```python
from build123d import *

# Parameters (mm, degrees)
SKETCH1_W           = 31.646470679
SKETCH1_H           = 16.00939105
BOSS_EXTRUDE1_DEPTH = 5
SKETCH1_3_W         = 65
SKETCH1_3_H         = 2.5
BOSS_EXTRUDE2_DEPTH = 20
SKETCH2_W           = 65
SKETCH2_H           = 2.5
BOSS_EXTRUDE3_DEPTH = 5
SKETCH2_3_W         = 65
SKETCH2_3_H         = 2.5
BOSS_EXTRUDE4_DEPTH = 7
SKETCH1_5_W         = 31.646470679
SKETCH1_5_H         = 16.00939105
BOSS_EXTRUDE5_DEPTH = 23
BOSS_EXTRUDE6_DEPTH = 16
BOSS_EXTRUDE7_DEPTH = 2
SKETCH5_W           = 9
SKETCH5_H           = 25
SKETCH5_W_2         = 5
SKETCH5_H_2         = 13.8


with BuildPart() as part:
    # Sketch1 → Boss-Extrude1 (new body)
    with BuildSketch(Plane.XY):
        with BuildLine():
            ThreePointArc((60, 43.75), (63.535533906, 42.285533906), (65, 38.75))
            Line((65, 38.75), (65, 7.5))
            Line((65, 7.5), (0, 7.5))
            Line((0, 7.5), (0, 38.75))
            ThreePointArc((0, 38.75), (1.464466094, 42.285533906), (5, 43.75))
            Line((5, 43.75), (60, 43.75))
        make_face()
        with Locations((31.682365604, 25.44274044)):
            Rectangle(SKETCH1_W, SKETCH1_H, mode=Mode.SUBTRACT)
        with Locations((31.682365604, 25.44274044)):
            Rectangle(SKETCH1_W, SKETCH1_H)
    extrude(amount=BOSS_EXTRUDE1_DEPTH)

    # Sketch1_3 → Boss-Extrude2 (add)
    with BuildSketch(Plane.XY):
        with Locations((32.5, 6.25)):
            Rectangle(SKETCH1_3_W, SKETCH1_3_H)
    extrude(amount=BOSS_EXTRUDE2_DEPTH)

    # Sketch2 → Boss-Extrude3 (add, symmetric)
    with BuildSketch(Plane.XY.offset(10)):
        with Locations((32.5, 3.75)):
            Rectangle(SKETCH2_W, SKETCH2_H)
    extrude(amount=BOSS_EXTRUDE3_DEPTH, both=True)

    # Sketch2_3 → Boss-Extrude4 (add, symmetric)
    with BuildSketch(Plane.XY.offset(10)):
        with Locations((32.5, 1.25)):
            Rectangle(SKETCH2_3_W, SKETCH2_3_H)
    extrude(amount=BOSS_EXTRUDE4_DEPTH, both=True)

    # Sketch1_5 → Boss-Extrude5 (add)
    with BuildSketch(Plane.XY):
        with Locations((31.682365604, 25.44274044)):
            Rectangle(SKETCH1_5_W, SKETCH1_5_H)
    extrude(amount=BOSS_EXTRUDE5_DEPTH)

    # Sketch3 → Boss-Extrude6 (add)
    with BuildSketch(Plane(origin=(0, 0, 0), x_dir=(-1, 0, 0), z_dir=(0, 0, -1))):
        with BuildLine():
            Line((-2, 33.67400262), (0, 33.67400262))
            Line((0, 33.67400262), (0, 38.75))
            ThreePointArc((0, 38.75), (-1.464466094, 42.285533906), (-5, 43.75))
            Line((-5, 43.75), (-60, 43.75))
            ThreePointArc((-60, 43.75), (-63.535533906, 42.285533906), (-65, 38.75))
            Line((-65, 38.75), (-65, 33.551986264))
            Line((-65, 33.551986264), (-63, 33.551986264))
            Line((-63, 33.551986264), (-63, 38.75))
            ThreePointArc((-63, 38.75), (-62.121320344, 40.871320344), (-60, 41.75))
            Line((-60, 41.75), (-5, 41.75))
            ThreePointArc((-5, 41.75), (-2.878679656, 40.871320344), (-2, 38.75))
            Line((-2, 38.75), (-2, 33.67400262))
        make_face()
        Polygon((-9.704230369, -9.009552441), (-4.852115184, -4.157437257), (-6.266328747, -2.743223694), (-10.532657494, -7.009552441), (-53.41460101, -7.009552441), (-57.531707428, -2.550119806), (-58.947047068, -3.965459446), (-54.290161463, -9.009552441), align=None)
    extrude(amount=BOSS_EXTRUDE6_DEPTH)


with BuildPart() as boss_extrude6_piece_1:
    # of the separate pieces the step leaves, piece 1, a body of its own (boss_extrude6_pieces)
    add(part.part.solids().sort_by_distance((65, 0, 3))[0])



with BuildPart() as boss_extrude6_piece_2:
    # of the separate pieces the step leaves, piece 2, a body of its own (boss_extrude6_pieces)
    add(part.part.solids().sort_by_distance((58.947047068, -3.965459446, 0))[0])


with BuildPart() as boss_extrude6_piece_1_1:
    add(boss_extrude6_piece_1.part)

    add(boss_extrude6_piece_2.part)  # Boss-Extrude7 merges Boss-Extrude6 piece 2
    # Sketch4 → Boss-Extrude7 (add)
    with BuildSketch(Plane(origin=(0, 0, -16), x_dir=(-1, 0, 0), z_dir=(0, 0, -1))):
        with BuildLine():
            Line((-60, 41.75), (-5, 41.75))
            ThreePointArc((-5, 41.75), (-2.878679656, 40.871320344), (-2, 38.75))
            Line((-2, 38.75), (-2, 33.67400262))
            Line((-2, 33.67400262), (0, 33.67400262))
            Line((0, 33.67400262), (0, 38.75))
            ThreePointArc((0, 38.75), (-1.464466094, 42.285533906), (-5, 43.75))
            Line((-5, 43.75), (-60, 43.75))
            ThreePointArc((-60, 43.75), (-63.535533906, 42.285533906), (-65, 38.75))
            Line((-65, 38.75), (-65, 33.551986264))
            Line((-65, 33.551986264), (-63, 33.551986264))
            Line((-63, 33.551986264), (-63, 38.75))
            ThreePointArc((-63, 38.75), (-62.121320344, 40.871320344), (-60, 41.75))
        make_face()
        with BuildLine():
            Line((-54.290161463, -9.009552441), (-9.704230369, -9.009552441))
            Line((-9.704230369, -9.009552441), (-4.852115184, -4.157437257))
            Line((-4.852115184, -4.157437257), (0, 0.694677928))
            Line((0, 0.694677928), (0, 33.67400262))
            Line((0, 33.67400262), (-2, 33.67400262))
            Line((-2, 33.67400262), (-2, 38.75))
            ThreePointArc((-2, 38.75), (-2.878679656, 40.871320344), (-5, 41.75))
            Line((-5, 41.75), (-60, 41.75))
            ThreePointArc((-60, 41.75), (-62.121320344, 40.871320344), (-63, 38.75))
            Line((-63, 38.75), (-63, 33.551986264))
            Line((-63, 33.551986264), (-65, 33.551986264))
            Line((-65, 33.551986264), (-65, 2.590780084))
            Line((-65, 2.590780084), (-58.947047068, -3.965459446))
            Line((-58.947047068, -3.965459446), (-54.290161463, -9.009552441))
        make_face()
    extrude(amount=BOSS_EXTRUDE7_DEPTH)

    # Sketch5 → Revolve1 (revolve)
    with BuildSketch(Plane.XY.offset(-6.5)):
        with Locations((28, 78.45)):
            Rectangle(SKETCH5_W, SKETCH5_H)
        Polygon((32.5, 57.55), (32.5, 65.95), (23.5, 65.95), (20.5, 65.95), (20.5, 57.55), (27.5, 57.55), align=None)
        with Locations((30, 50.65)):
            Rectangle(SKETCH5_W_2, SKETCH5_H_2)
    revolve(axis=Axis((32.5, 92.408225654, -6.5), (0, -1, 0)))


solid = boss_extrude6_piece_1_1.part
```
Part model, mm, in its own coordinate system. A direction names the side the tool comes from. Round coordinates to 2 decimals unless told otherwise and drop trailing zeros. Loops run counter-clockwise (first coordinate to the right, second up) from the corner with the lowest first, then second, coordinate; pieces in that order, holes last.
1. Drill centre lines: line 1 along Y through (x, z) = (53, -7); line 2 along Z through (x, y) = (29, 6); line 3 along Z through (x, y) = (6.5, 11.5). Where is each one in solid material? Low to high.
Solutions:
line 1: y = -9.01 to -7.01, 41.75 to 43.75
line 2: z = -18 to -16, 0 to 20
line 3: z = -18 to -16, 0 to 5
2. Two-plate mould, pull along Y, no slides. Class faces 5 (the face through (65, 21, 1)), 6 (the face through (33, 90.95, -7)), 7 (the face through (32, 5, 2)), 8 (the face through (55.444, -4.811, -7.888)): pulls with the +Y half, pulls with the -Y half, needs draft (parallel to the pull), parting line crosses it, or undercut.
Solutions:
face 5: needs draft
face 6: pulls with the +Y half
face 7: undercut
face 8: undercut
3. Slice it at C-C (y = 67). Give the cut face in (x, z), and give its area (3 significant figures).
Solutions:
outline: circle Ø18 at (32.5, -6.5)
area: 254 mm2
4. Flat gauge pins, fed straight in: pin 1 (1 mm diameter, centred on y = 66.5, z = -4.5, fed in from -X); pin 2 (18.5 mm diameter, centred on x = 34.5, y = 21.5, fed in from -Z); pin 3 (4 mm diameter, centred on y = 79.5, z = 3, fed in from -X). Where does each tip first touch, or does it go through?
Solutions:
pin 1: stops at x = 23.63
pin 2: stops at z = -18
pin 3: stops at x = 27.53
5. Slice it at B-B (z = 7). Give the cut face in (x, y), and give its area (3 significant figures).
Solutions:
outline: (0, 0) - (65, 0) - (65, 7.5) - (0, 7.5) - close; (15.86, 17.44) - (47.51, 17.44) - (47.51, 33.45) - (15.86, 33.45) - close
area: 994 mm2
6. 3-axis set-ups, long thin cutter, end or side, ignore diameter. For faces 1 (the face through (32, 0, 10)), 2 (the face through (32, -7.01, -8)), 3 (the face through (21.415, 61.691, -1.904)), 4 (the face through (32, 7.5, 12)): which of +Z, -Z, +X, -X, +Y, -Y reach the whole face in a straight line?
Solutions:
face 1: +Z, +X, -X, -Y
face 2: +Z
face 3: +Y
face 4: +Z, +X, -X
